Source: CAD feature listing. Evaluate the final solid. Frame: model axes, mm. Round coordinates to 2 decimals unless told otherwise and drop trailing zeros. Order: outer loops, then holes, each group sorted by start corner. A loop starts at its lowest first (then second) coordinate and runs counter-clockwise, first axis right, second up.
```python
from build123d import *

# Parameters (mm, degrees)
SKETCH1_W           = 711.2
SKETCH1_H           = 419.1
BOSS_EXTRUDE1_DEPTH = 2.54
CUT_EXTRUDE1_DEPTH  = 413.757815311


with BuildPart() as part:
    # Sketch1 → Boss-Extrude1 (new body)
    with BuildSketch(Plane(origin=(0, 0, 0), x_dir=(0, 1, 0), z_dir=(0, 0, 1))):
        Rectangle(SKETCH1_W, SKETCH1_H)
    extrude(amount=BOSS_EXTRUDE1_DEPTH)

    # Sketch2 → Cut-Extrude1 (cut, through all)
    with BuildSketch(Plane.XY.offset(2.54)):
        Polygon((-144.11270055, 165.1), (-19.05, 290.16270055), (-19.05, 355.6), (-209.55, 355.6), (-209.55, 165.1), align=None)
        Polygon((-19.05, -355.6), (-209.55, -355.6), (-209.55, -165.1), (-144.11270055, -165.1), (-19.05, -290.16270055), align=None)
    extrude(amount=-CUT_EXTRUDE1_DEPTH, mode=Mode.SUBTRACT)


solid = part.part
```
1. Section A-A on z = 0.75. Return loops of the section in (x, y), plus the area to 3 significant figures.
2. Section B-B on x = -168. Return loops of the section in (y, z).
3. Section C-C on y = -224.5. Return loops of the section in (x, z), plus the area to 3 significant figures.
4. Pull-direction query (Y, two-part tool) for faces 1 (the face through (-82.457, 226.756, 1.288)), 2 (the face through (44, -5, 0)), 3 (the face through (-82.457, -226.756, 1.288)); classes: released by +Y, released by -Y, zero draft, split by the parting line, or undercut.
5. First-contact query: pin 1 (0.8 mm diameter, centred on x = -173, z = 1.5, fed in from -Y); pin 2 (1 mm diameter, centred on x = 7.5, y = -137.5, fed in from -Z). Flat tips, straight axial feed; report the tip coordinate or a pass-through.
6. Line query: line 1 along X through (y, z) = (300.5, 0.2); line 2 along Y through (x, z) = (-171.5, 0.1); line 3 along X through (y, z) = (277, 2.1). Output: solid intervals per line, ascending.
Result:
1. outline: (-209.55, -165.1) - (-144.11, -165.1) - (-19.05, -290.16) - (-19.05, -355.6) - (209.55, -355.6) - (209.55, 355.6) - (-19.05, 355.6) - (-19.05, 290.16) - (-144.11, 165.1) - (-209.55, 165.1) - close
1. area: 241,000 mm2
2. outline: (-165.1, 0) - (165.1, 0) - (165.1, 2.54) - (-165.1, 2.54) - close
3. outline: (-84.71, 0) - (209.55, 0) - (209.55, 2.54) - (-84.71, 2.54) - close
3. area: 747 mm2
4. face 1: released by +Y
4. face 2: zero draft
4. face 3: released by -Y
5. pin 1: stops at y = -165.1
5. pin 2: stops at z = 0
6. line 1: x = -19.05 to 209.55
6. line 2: y = -165.1 to 165.1
6. line 3: x = -32.21 to 209.55
